```python
from build123d import *

# Parameters (mm, degrees)
SKETCH1_R           = 4.7625
BOSS_EXTRUDE1_DEPTH = 1.5875
SKETCH2_R           = 1.5875
CUT_EXTRUDE1_DEPTH  = 74.611450938
FILLET1_R           = 0.2
FILLET2_R           = 0.2


with BuildPart() as part:
    # Sketch1 → Boss-Extrude1 (new body)
    with BuildSketch(Plane.XY):
        with Locations((68.398246491, 3.214386977)):
            Circle(SKETCH1_R)
    extrude(amount=BOSS_EXTRUDE1_DEPTH)

    # Sketch2 → Cut-Extrude1 (cut, through all)
    with BuildSketch(Plane(origin=(0, 0, 0), x_dir=(-1, 0, 0), z_dir=(0, 0, -1))):
        with Locations((-68.398246491, 3.214386977)):
            Circle(SKETCH2_R)
    extrude(amount=-CUT_EXTRUDE1_DEPTH, mode=Mode.SUBTRACT)

    # Fillet1
    fillet1_edges = [part.edges().sort_by_distance(p)[0] for p in [
        (63.635746491, 3.214386977, 1.5875),
        (69.985746491, 3.214386977, 1.5875),
        (69.985746491, 3.214386977, 0),
    ]]
    fillet(fillet1_edges, radius=FILLET1_R)

    # Fillet2
    fillet2_edges = [part.edges().sort_by_distance(p)[0] for p in [
        (63.635746491, 3.214386977, 0),
    ]]
    fillet(fillet2_edges, radius=FILLET2_R)


solid = part.part
```
CAD build for the part. Positions are in the model's coordinates, mm. Give positions to 0.01 mm unless a question says otherwise; leave off trailing zeros. Order: outer loops, then holes, each group sorted by start corner. A loop starts at its lowest first (then second) coordinate and runs counter-clockwise, first axis right, second up. Notation, with made-up numbers: M 27.5,-17 L 45.5,-17 A11 ccw 45.5,-2 Z; hole C 88,37 d7. An arc over 180 degrees is marked long. Put each result on its own line as item: value. Start each with the question number.
(1) Mould opens along Y. For faces 1 (the flat face through (68, 1, 0)), 2 (the cylindrical face through (72.8, 1.4, 0.8)), 3 (the cylindrical face through (69.568, 4.287, 0.785)) say: +Y half, -Y half, draft (parallel to the pull), parting line (faces both ways), or undercut.
(2) Saw through at A-A, the plane z = 1. Write the cut outline in (x, y) (1 decimal), then the cut area to 3 significant figures.
(3) Drill centre lines: line 1 along Y through (x, z) = (67, 1.25); line 2 along X through (y, z) = (3.5, 1.5); line 3 along X through (y, z) = (2.5, 0.6). Where is each one in solid material? Low to high.
Check result:
1. face 1: draft
1. face 2: parting line
1. face 3: undercut
2. outline: C 68.4,3.2 d9.5; hole C 68.4,3.2 d3.2
2. area: 63.3 mm2
3. line 1: y = -1.34 to 2.46, 3.97 to 7.77
3. line 2: x = 63.68 to 66.8, 70 to 73.12
3. line 3: x = 63.69 to 66.98, 69.82 to 73.11
